Part model, mm, in its own coordinate system. A direction names the side the tool comes from. Coordinates: 2 decimals unless noted, no trailing zeros. Order: outer loops, then holes, each group sorted by start corner. A loop starts at its lowest first (then second) coordinate and runs counter-clockwise, first axis right, second up. Notation, with made-up numbers: (-10.75, 70.5) - (27.25, 70.5) arc R17 ccw to (27.25, 94.5) - close; hole circle Ø11 at (58, 65). An arc over 180 degrees is marked (long way). Use a Markdown table: item, result. Add a question column.
1) Two-plate mould, pull along Z, no slides. Class faces 1 (the face through (149, 0, -150.804)), 2 (the face through (-4, 12.7, 7)), 3 (the face through (-153, 0, -150.804)), 4 (the face through (-1, -1, -233.354)): +Z half, -Z half, draft (parallel to the pull), parting line (faces both ways), or undercut.
2) Wall check: L1, parallel to Z at x = -71, y = 7; L2, parallel to Y at x = 52.5, z = 52; L3, parallel to X at y = -3, z = -206.5 (3 decimals). Give the ranges that are in metal, low to high. Write a range as [from, to].
3) Tool access for faces 5 (the face through (22.225, 0, -189)), 6 (the face through (-4, -12.7, 7)), 7 (the face through (-22.225, 0, -189)): list every direction of +Z, -Z, +X, -X, +Y, -Y with a clear straight run to the whole face (end or side of a thin tool).
4) Saw through at D-D on z = -168. List the corners of the cut face in (x, y) (3 decimals), then the cut area to 3 significant figures.
5) Saw through at B-B on y = 0. List the corners of the cut face in (x, z) (3 decimals), then the cut area to 3 significant figures.
6) Saw through at A-A on x = 0. List the corners of the cut face in (y, z), then the cut area to 3 significant figures.
7) Drop flat-ended pins along their axis: P1, Ø12.5, axis at x = -210.5, y = -4.5, coming from the -Z side; P2, Ø20.5, axis at y = -6.5, z = -187, coming from the -X side (3 decimals); P3, Ø3, axis at x = -51.5, y = 64, coming from the +Z side. Give the stop position or say it passes through.
8) Saw through at C-C on z = -129. List the corners of the cut face in (x, y).
```python
from build123d import *

# Parameters (mm, degrees)
F0_W     = 44.45
F0_H     = 76.2
F1_DEPTH = 12.7
F2_R     = 101.6
F3_DEPTH = 6.35


with BuildPart() as f1:
    # F0 (on Front) → F1 (new body, symmetric)
    with BuildSketch(Plane.XZ):
        Polygon((279.4, -150.804145), (279.4, 150.804145), (-279.4, 150.804145), align=None)
        Polygon((279.4, -150.804145), (-279.4, 150.804145), (-279.4, -150.804145), (-22.225, -150.804145), (22.225, -150.804145), align=None)
        with Locations((0, -188.904145)):
            Rectangle(F0_W, F0_H)
    extrude(amount=F1_DEPTH, both=True)

    # F2 (on face) → F3 (join)
    with BuildSketch(Plane(origin=(0, 0, -227.004145), x_dir=(1, 0, 0), z_dir=(0, 0, -1))):
        Circle(F2_R)
    extrude(amount=F3_DEPTH)


solid = f1.part
```
Results are:
| question | item | result |
|---|---|---|
| 1 | face 1 | undercut |
| 1 | face 2 | draft |
| 1 | face 3 | undercut |
| 1 | face 4 | -Z half |
| 2 | L1 | [-233.35, -227], [-150.8, 150.8] |
| 2 | L2 | [-12.7, 12.7] |
| 2 | L3 | [-22.225, 22.225] |
| 3 | face 5 | +X, +Y, -Y |
| 3 | face 6 | +Z, +X, -X, -Y |
| 3 | face 7 | -X, +Y, -Y |
| 4 | outline | (-22.225, -12.7) - (22.225, -12.7) - (22.225, 12.7) - (-22.225, 12.7) - close |
| 4 | area | 1,130 mm2 |
| 5 | outline | (-279.4, -150.804) - (-22.225, -150.804) - (-22.225, -227.004) - (-101.6, -227.004) - (-101.6, -233.354) - (101.6, -233.354) - (101.6, -227.004) - (22.225, -227.004) - (22.225, -150.804) - (279.4, -150.804) - (279.4, 150.804) - (-279.4, 150.804) - close |
| 5 | area | 173,000 mm2 |
| 6 | outline | (-101.6, -233.35) - (101.6, -233.35) - (101.6, -227) - (12.7, -227) - (12.7, 150.8) - (-12.7, 150.8) - (-12.7, -227) - (-101.6, -227) - close |
| 6 | area | 10,900 mm2 |
| 7 | P1 | z = -150.8 |
| 7 | P2 | x = -22.225 |
| 7 | P3 | z = -227 |
| 8 | outline | (-279.4, -12.7) - (279.4, -12.7) - (279.4, 12.7) - (-279.4, 12.7) - close |
